Part model, mm, in its own coordinate system. Face numbers are marked on the shaded views. A direction names the side the tool comes from. Coordinates: 2 decimals unless noted, no trailing zeros. Order: outer loops, then holes, each group sorted by start corner. A loop starts at its lowest first (then second) coordinate and runs counter-clockwise, first axis right, second up.
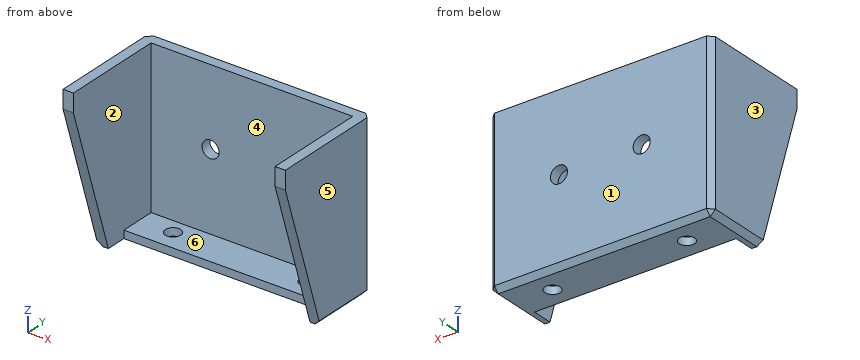
```python
from build123d import *

# Parameters (mm, degrees)
SKETCH_1_W          = 43
SKETCH_1_H          = 31.5
EXTRUDE_1_DEPTH     = 2
SKETCH_4_W          = 2
SKETCH_4_H          = 31.5
EXTRUDE_3_DEPTH     = 20
SKETCH_7_W          = 39
SKETCH_7_H          = 1.5
EXTRUDE_4_DEPTH     = 11
SKETCH_6_R          = 1.65
CUT_EXTRUDE_2_DEPTH = 12
SKETCH_5_R          = 1.5
CUT_EXTRUDE_1_DEPTH = 12
CHAMFER_1_SIZE      = 1
CUT_EXTRUDE_4_DEPTH = 50
SKETCH_13_W         = 39
SKETCH_13_H         = 4
CUT_EXTRUDE_8_DEPTH = 10


with BuildPart() as part:
    # 草图1 → 凸台-拉伸1 (new body)
    with BuildSketch(Plane(origin=(0, 0, 0), x_dir=(1, 0, 0), z_dir=(0, 1, 0))):
        with Locations((0, -5.266908213)):
            Rectangle(SKETCH_1_W, SKETCH_1_H)
    extrude(amount=EXTRUDE_1_DEPTH)

    # 草图4 → 凸台-拉伸3 (add)
    with BuildSketch(Plane.XZ):
        with Locations((-20.5, 5.266908213)):
            Rectangle(SKETCH_4_W, SKETCH_4_H)
        with Locations((20.5, 5.266908213)):
            Rectangle(SKETCH_4_W, SKETCH_4_H)
    extrude(amount=EXTRUDE_3_DEPTH)

    # 草图7 → 凸台-拉伸4 (add)
    with BuildSketch(Plane.XZ):
        with Locations((0, -9.733091787)):
            Rectangle(SKETCH_7_W, SKETCH_7_H)
    extrude(amount=EXTRUDE_4_DEPTH)

    # 草图6 → 切除-拉伸2 (cut)
    with BuildSketch(Plane.XZ):
        with Locations(Location((8, 6.016908213, 0), (0, 0, 270))):
            Circle(SKETCH_6_R)
        with Locations(Location((-8, 6.016908213, 0), (0, 0, 270))):
            Circle(SKETCH_6_R)
    extrude(amount=-CUT_EXTRUDE_2_DEPTH, mode=Mode.SUBTRACT)

    # 草图5 → 切除-拉伸1 (cut)
    with BuildSketch(Plane(origin=(0, 0, -10.483091787), x_dir=(-1, 0, 0), z_dir=(0, 0, -1))):
        with Locations((-13, -3)):
            Circle(SKETCH_5_R)
        with Locations((13, -3)):
            Circle(SKETCH_5_R)
    extrude(amount=-CUT_EXTRUDE_1_DEPTH, mode=Mode.SUBTRACT)

    # 倒角1
    chamfer_1_edges = [part.edges().sort_by_distance(p)[0] for p in [
        (21.5, 2, 5.266908213),
        (0, 2, -10.483091787),
        (-21.5, 2, 5.266908213),
        (-21.5, -9, -10.483091787),
        (21.5, -9, -10.483091787),
    ]]
    chamfer(chamfer_1_edges, length=CHAMFER_1_SIZE)

    # 草图10 → 切除-拉伸4 (cut, symmetric)
    with BuildSketch(Plane(origin=(-19.5, 0, 0), x_dir=(0, 0, -1), z_dir=(1, 0, 0))):
        Polygon((10.483091787, -20), (10.483091787, -11), (-17.516908213, -20), align=None)
    extrude(amount=CUT_EXTRUDE_4_DEPTH, both=True, mode=Mode.SUBTRACT)

    # 草图13 → 切除-拉伸8 (cut)
    with BuildSketch(Plane(origin=(0, 0, -10.483091787), x_dir=(-1, 0, 0), z_dir=(0, 0, -1))):
        with Locations((0, -9)):
            Rectangle(SKETCH_13_W, SKETCH_13_H)
    extrude(amount=-CUT_EXTRUDE_8_DEPTH, mode=Mode.SUBTRACT)


solid = part.part
```
(1) Drop flat-ended pins along their axis: pin 1 (3.5 mm diameter, centred on x = 2, y = -3, fed in from +Z); pin 2 (12 mm diameter, centred on x = 6.5, z = 2.5, fed in from -Y). Give the stop position or say it passes through.
(2) Slice it at A-A, the plane x = 13. Give the cut face in (y, z), then the cut area to 3 significant figures.
(3) Tool access for the marked faces 1 and 2: list every direction of +Z, -Z, +X, -X, +Y, -Y with a clear straight run to the whole face (end or side of a thin tool).
(4) Slice it at B-B, the plane y = -9.75. Give the cut face in (x, z), then the cut area to 3 significant figures.
(5) Slice it at C-C, the plane x = -8. Give the cut face in (y, z).
(6) Pull direction X, two halves, no side cores. Call the marked faces 3, 4, 5 and 6: +X half, -X half, draft (parallel to the pull), parting line (faces both ways), or undercut.
(7) Slice it at D-D, the plane y = -5.5. Give the cut face in (x, z).
(8) Probe line 1 (X direction, y = -12.75, z = 14); line 2 (Y direction, x = 16, z = 0); line 3 (Z direction, x = 17, y = -4). List the from-to ranges inside material, lowest first.
Here are the results:
1. pin 1: stops at z = -8.98
1. pin 2: stops at y = 0
2. outline: (-7, -10.48) - (-4.5, -10.48) - (-4.5, -8.98) - (-7, -8.98) - close; (-1.5, -10.48) - (1, -10.48) - (2, -9.48) - (2, 21.02) - (0, 21.02) - (0, -8.98) - (-1.5, -8.98) - close
2. area: 68.5 mm2
3. face 1: +Z, -Z, +X, -X, +Y
3. face 2: +Z, -Y
4. outline: (-21.5, -9.48) - (-20.5, -10.48) - (-19.5, -10.48) - (-19.5, 21.02) - (-21.5, 21.02) - close; (19.5, -10.48) - (20.5, -10.48) - (21.5, -9.48) - (21.5, 21.02) - (19.5, 21.02) - close
4. area: 125 mm2
5. outline: (-7, -10.48) - (1, -10.48) - (2, -9.48) - (2, 4.37) - (0, 4.37) - (0, -8.98) - (-7, -8.98) - close; (0, 7.67) - (2, 7.67) - (2, 21.02) - (0, 21.02) - close
6. face 3: -X half
6. face 4: undercut
6. face 5: +X half
6. face 6: undercut
7. outline: (-21.5, -9.48) - (-20.5, -10.48) - (20.5, -10.48) - (21.5, -9.48) - (21.5, 21.02) - (19.5, 21.02) - (19.5, -8.98) - (-19.5, -8.98) - (-19.5, 21.02) - (-21.5, 21.02) - close
8. line 1: x = -21.5 to -19.5, 19.5 to 21.5
8. line 2: y = 0 to 2
8. line 3: z = -10.48 to -8.98
